For this review, take the finished solid that the model builds, in its own axes (mm). A direction names the side the tool comes from. Round coordinates to 2 decimals unless told otherwise and drop trailing zeros. Order: outer loops, then holes, each group sorted by start corner. A loop starts at its lowest first (then second) coordinate and runs counter-clockwise, first axis right, second up. Notation, with made-up numbers: (55, -34) -> (95, -34) arc R9 cw to (95, -22) -> close; hole circle Ø2 at (10, 63.25). An arc over 180 degrees is marked (long way). Use a Markdown table: item, result. Add a question column.
1) Clearance check with flat-ended pins moving along their axes: P1, Ø3, axis at y = -7, z = 33, coming from the +X side; P2, Ø3, axis at y = -5.5, z = 33, coming from the -X side; P3, Ø7, axis at x = 6.5, y = -8, coming from the +Z side. State where each tip first meets the part, or that it passes through.
2) Wall thickness on line 1 along Y through (x, z) = (88, 7.75); line 2 along X through (y, z) = (-9, 35); line 3 along X through (y, z) = (-11.5, 14): over which ranges is each line inside the solid? List them lowest first. Write a range as [from, to].
3) Draft analysis for pull direction X (two halves, no side actions). For faces 4 (the face through (0, 0, 5)), 5 (the face through (39, 0, 43)), 6 (the face through (51, -20, 19)), state which applies: pulls with the +X half, pulls with the -X half, needs draft (parallel to the pull), parting line crosses it, or undercut.
4) Consider section B-B (x = 80). State the section outline as (y, z) points, plus the area to 3 significant figures.
5) Consider section C-C (z = 9). State the section outline as (x, y) points, plus the area to 3 significant figures.
6) Consider section A-A (y = 0). State the section outline as (x, z) points.
7) Machinability: for faces 1 (the face through (76, 0, 30)), 2 (the face through (24, 0, 30)), 3 (the face through (53, 0, 32)), which of the approach directions +Z, -Z, +X, -X, +Y, -Y give a long, thin tool a straight path to every point of the face, cutting with its end or side? Answer none if there is none.
8) Consider section D-D (y = 15.5). State the section outline as (x, z) points.
Solid Edge part; units mm, degrees
sketch "Sketch1" plane through (0, 0, 0) normal (0, -1, 0) x (1, 0, 0)
  line L0 (32, 50) -> (47, 35)
  line L1 (47, 29) -> (47, 35)
  line L2 (53, 29) -> (47, 29)
  line L3 (53, 35) -> (53, 29)
  line L4 (53, 35) -> (68, 50)
  line L5 (76, 50) -> (68, 50)
  line L6 (76, 10) -> (76, 50)
  line L7 (100, 10) -> (76, 10)
  line L8 (100, 0) -> (100, 10)
  line L9 (0, 0) -> (100, 0)
  line L10 (0, 0) -> (0, 10)
  line L11 (0, 10) -> (24, 10)
  line L12 (24, 10) -> (24, 50)
  line L13 (24, 50) -> (32, 50)
extrude "ExtrudedProtrusion_1" add sketch "Sketch1" against normal blind 20 and the other way blind 20
sketch "Sketch2" plane through (88, 0, 10) normal (0, 0, 1) x (1, 0, 0)
  circle A0 centre (0, 0) radius 10
extrude "ExtrudedCutout_1" cut sketch "Sketch2" against normal blind 10
Results list:
| question | item | result |
|---|---|---|
| 1 | P1 | x = 76 |
| 1 | P2 | x = 24 |
| 1 | P3 | z = 10 |
| 2 | line 1 | [-20, -10], [10, 20] |
| 2 | line 2 | [24, 47], [53, 76] |
| 2 | line 3 | [24, 76] |
| 3 | face 4 | pulls with the -X half |
| 3 | face 5 | undercut |
| 3 | face 6 | needs draft |
| 4 | outline | (-20, 0) -> (-6, 0) -> (-6, 10) -> (-20, 10) -> close; (6, 0) -> (20, 0) -> (20, 10) -> (6, 10) -> close |
| 4 | area | 280 mm2 |
| 5 | outline | (0, -20) -> (100, -20) -> (100, 20) -> (0, 20) -> close; hole circle Ø20 at (88, 0) |
| 5 | area | 3,690 mm2 |
| 6 | outline | (0, 0) -> (78, 0) -> (78, 10) -> (76, 10) -> (76, 50) -> (68, 50) -> (53, 35) -> (53, 29) -> (47, 29) -> (47, 35) -> (32, 50) -> (24, 50) -> (24, 10) -> (0, 10) -> close; (98, 0) -> (100, 0) -> (100, 10) -> (98, 10) -> close |
| 7 | face 1 | +Z, +X, +Y, -Y |
| 7 | face 2 | +Z, -X, +Y, -Y |
| 7 | face 3 | +Z, +Y, -Y |
| 8 | outline | (0, 0) -> (100, 0) -> (100, 10) -> (76, 10) -> (76, 50) -> (68, 50) -> (53, 35) -> (53, 29) -> (47, 29) -> (47, 35) -> (32, 50) -> (24, 50) -> (24, 10) -> (0, 10) -> close |
